from build123d import *

# Parameters (mm, degrees)
F1_DEPTH = 3.175
F2_DEPTH = 5.08


with BuildPart() as f1:
    # F0 (on Top) → F1 (new body)
    with BuildSketch(Plane.XY):
        with BuildLine():
            Line((6.8534065496, 13.273686968), (-9.0469934504, 13.273686968))
            Line((-9.0469934504, 13.273686968), (-3.2091541804, 10.354767333))
            ThreePointArc((-3.2091541804, 10.354767333), (-0.5541880245, 11.5971004374), (1.2648976422, 9.298586968))
            ThreePointArc((1.2648976422, 9.298586968), (1.2017200189, 8.7559815421), (1.0155672796, 8.2424066031))
            Line((1.0155672796, 8.2424066031), (6.8534065496, 5.323486968))
            Line((6.8534065496, 5.323486968), (6.8534065496, 13.273686968))
        make_face()
        with BuildLine():
            Line((-3.2091541804, 10.354767333), (-9.0469934504, 13.273686968))
            Line((-9.0469934504, 13.273686968), (-9.0469934504, 5.323486968))
            Line((-9.0469934504, 5.323486968), (6.8534065496, 5.323486968))
            Line((6.8534065496, 5.323486968), (1.0155672796, 8.2424066031))
            ThreePointArc((1.0155672796, 8.2424066031), (-2.1529738154, 7.1862262381), (-3.2091541804, 10.354767333))
        make_face()
        with BuildLine():
            ThreePointArc((1.2648976422, 9.298586968), (-0.5541880245, 11.5971004374), (-3.2091541804, 10.354767333))
            Line((-3.2091541804, 10.354767333), (1.0155672796, 8.2424066031))
            ThreePointArc((1.0155672796, 8.2424066031), (1.2017200189, 8.7559815421), (1.2648976422, 9.298586968))
        make_face()
        with BuildLine():
            Line((1.0155672796, 8.2424066031), (-3.2091541804, 10.354767333))
            ThreePointArc((-3.2091541804, 10.354767333), (-2.1529738154, 7.1862262381), (1.0155672796, 8.2424066031))
        make_face()
    extrude(amount=F1_DEPTH)

    # F0 (on Top) → F2 (join)
    with BuildSketch(Plane.XY):
        with BuildLine():
            ThreePointArc((1.2648976422, 9.298586968), (-0.5541880245, 11.5971004374), (-3.2091541804, 10.354767333))
            Line((-3.2091541804, 10.354767333), (1.0155672796, 8.2424066031))
            ThreePointArc((1.0155672796, 8.2424066031), (1.2017200189, 8.7559815421), (1.2648976422, 9.298586968))
        make_face()
        with BuildLine():
            Line((1.0155672796, 8.2424066031), (-3.2091541804, 10.354767333))
            ThreePointArc((-3.2091541804, 10.354767333), (-2.1529738154, 7.1862262381), (1.0155672796, 8.2424066031))
        make_face()
    extrude(amount=F2_DEPTH)


solid = f1.part
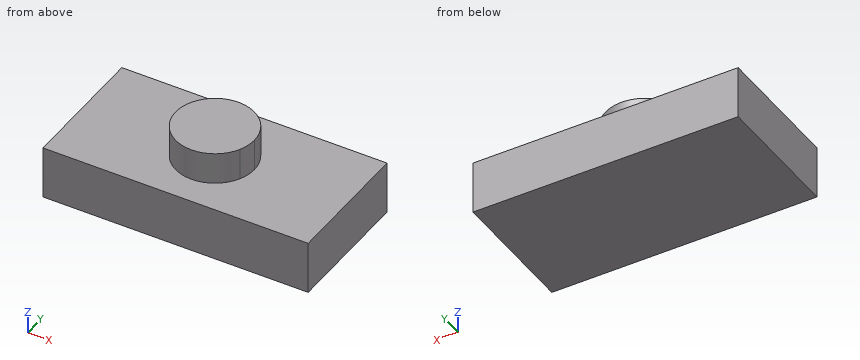
Build history of the part. All positions in model axes, mm. Coordinates: 2 decimals unless noted, no trailing zeros. Write each loop counter-clockwise with the first axis right and the second up, starting at its lowest first coordinate (ties: lowest second). Pieces come first, ordered by that corner, then holes.
(1) Pin check, flat tip, straight feed: pin 1 Ø2 at (x, y) = (-3.5, 6.5) entering from +Z (3 decimals). Stop position of the tip, or through.
(2) Cut at C-C on z = 4.3. List the corners of the cut face in (x, y).
(3) Cut at A-A on x = -1. List the corners of the cut face in (y, z) (3 decimals).
(4) Cut at B-B on y = 11.25. List the corners of the cut face in (x, z) (3 decimals), and give its area (3 significant figures).
(5) Drill centre lines: line 1 (Z direction, x = 2.75, y = 7.25) (3 decimals); line 2 (Y direction, x = -0.5, z = 4.45); line 3 (Y direction, x = 0.5, z = 4.85). Where is each one in solid material? Low to high.
(6) Cut at D-D on x = -8. List the corners of the cut face in (y, z) (3 decimals).
Working result:
1. pin 1: stops at z = 3.175
2. outline: circle Ø4.72 at (-1.1, 9.3)
3. outline: (5.323, 0) - (13.274, 0) - (13.274, 3.175) - (11.658, 3.175) - (11.658, 5.08) - (6.939, 5.08) - (6.939, 3.175) - (5.323, 3.175) - close
4. outline: (-9.047, 0) - (6.853, 0) - (6.853, 3.175) - (0.233, 3.175) - (0.233, 5.08) - (-2.427, 5.08) - (-2.427, 3.175) - (-9.047, 3.175) - close
4. area: 55.6 mm2
5. line 1: z = 0 to 3.175
5. line 2: y = 7.01 to 11.58
5. line 3: y = 7.56 to 11.04
6. outline: (5.323, 0) - (13.274, 0) - (13.274, 3.175) - (5.323, 3.175) - close
